```python
from build123d import *

# Parameters (mm, degrees)
F0_W     = 25
F0_H     = 34.675
F0_W_2   = 15.7
F0_H_2   = 27.7
F0_R     = 4.075
F1_DEPTH = 25
F2_R     = 10
F3_R     = 1


with BuildPart() as f1:
    # F0 (on Top) → F1 (new body)
    with BuildSketch(Plane.XY):
        with Locations((0.225, -0.0875)):
            Rectangle(F0_W, F0_H)
        Rectangle(F0_W_2, F0_H_2, mode=Mode.SUBTRACT)
        with BuildLine():
            Line((-12.275, 17.25), (12.725, 17.25))
            Line((12.725, 17.25), (8.530193, 31.366524))
            ThreePointArc((8.530193, 31.366524), (0, 22.836331), (-8.530193, 31.366524))
            Line((-8.530193, 31.366524), (-12.275, 17.25))
        make_face()
        with BuildLine():
            ThreePointArc((-8.530193, 31.366524), (0, 22.836331), (8.530193, 31.366524))
            ThreePointArc((8.530193, 31.366524), (0, 39.896717), (-8.530193, 31.366524))
        make_face()
        with Locations((0, 31.366524)):
            Circle(F0_R, mode=Mode.SUBTRACT)
    extrude(amount=F1_DEPTH)

    # F2
    f2_edges = [f1.edges().sort_by_distance(p)[0] for p in [
        (12.725, 17.25, 12.5),
        (8.530193, 31.366524, 12.5),
        (-8.530193, 31.366524, 12.5),
        (-12.275, 17.25, 12.5),
    ]]
    fillet(f2_edges, radius=F2_R)

    # F3
    f3_edges = [f1.edges().sort_by_distance(p)[0] for p in [
        (12.725, -0.814676, 25),
        (12.620892, 17.234859, 25),
        (0.225, -17.425, 25),
        (10.587354, 24.443688, 25),
        (-12.275, -0.739421, 25),
        (8.631638, 31.192913, 25),
        (-12.191068, 17.239057, 25),
        (-0.040943, 39.896618, 25),
        (-10.370209, 24.430349, 25),
        (-8.612072, 31.208214, 25),
        (7.85, 0, 25),
        (0, -13.85, 25),
        (-7.85, 0, 25),
        (0, 13.85, 25),
        (-4.075, 31.366524, 25),
    ]]
    fillet(f3_edges, radius=F3_R)


solid = f1.part
```
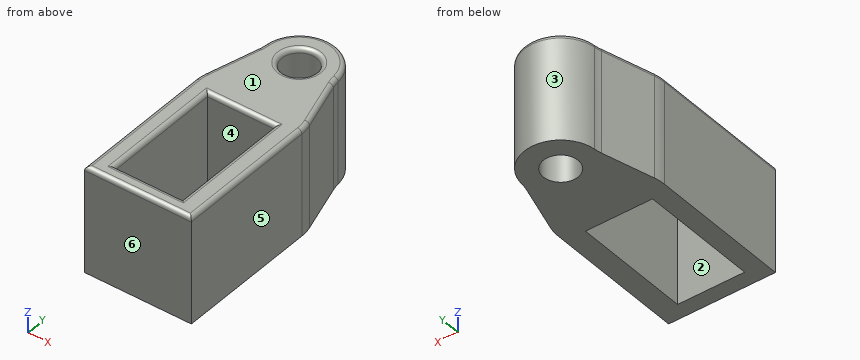
Part model, mm, in its own coordinate system. Face numbers are marked on the shaded views. A direction names the side the tool comes from. Round coordinates to 2 decimals unless told otherwise and drop trailing zeros. Loops run counter-clockwise (first coordinate to the right, second up) from the corner with the lowest first, then second, coordinate; pieces in that order, holes last.
1. Drill centre lines: line 1 along Y through (x, z) = (0, 6.25) (3 decimals); line 2 along X through (y, z) = (13.5, 13.5) (3 decimals); line 3 along Y through (x, z) = (-3.75, 13.5) (3 decimals). Where is each one in solid material? Low to high.
Solutions:
line 1: y = -17.425 to -13.85, 13.85 to 27.292, 35.442 to 39.897
line 2: x = -12.275 to -7.85, 7.85 to 12.725
line 3: y = -17.425 to -13.85, 13.85 to 29.772, 32.961 to 39.028
2. Flat gauge pins, fed straight in: pin 1 (5 mm diameter, centred on x = 4.5, z = 3.5, fed in from +Y); pin 2 (1 mm diameter, centred on x = -3.5, z = 21.5, fed in from +Y); pin 3 (4 mm diameter, centred on y = 21.5, z = 13, fed in from -X); pin 4 (8 mm diameter, centred on x = 1, y = -7, fed in from +Z). Where does each tip first touch, or does it go through?
Solutions:
pin 1: stops at y = 39.66
pin 2: stops at y = 39.35
pin 3: stops at x = -11.68
pin 4: passes through
3. 3-axis set-ups, long thin cutter, end or side, ignore diameter. For the marked faces 1 and 2: which of +Z, -Z, +X, -X, +Y, -Y reach the whole face in a straight line?
Solutions:
face 1: +Z, +X, -X, +Y, -Y
face 2: +Z, -Z
4. Two-plate mould, pull along Y, no slides. Class the marked faces 3, 4, 5 and 6: pulls with the +Y half, pulls with the -Y half, needs draft (parallel to the pull), parting line crosses it, or undercut.
Solutions:
face 3: pulls with the +Y half
face 4: undercut
face 5: needs draft
face 6: pulls with the -Y half
5. Slice it at C-C (x = 3.5). Count the separate pieces of the cut face and the enclosed holes in it, and give its area (3 significant figures).
Solutions:
separate pieces: 3
enclosed holes: 0
area: 616 mm2
6. Slice it at B-B (z = 4.5). Give the cut face in (x, y) (3 decimals).
Solutions:
outline: (-12.275, -17.425) - (12.725, -17.425) - (12.725, 15.796) arc R10 ccw to (12.311, 18.644) - (8.864, 30.243) arc R10 cw to (8.493, 32.161) arc R8.53 ccw to (-8.5, 32.079) arc R10 cw to (-8.8, 30.35) - (-11.941, 18.51) arc R10 ccw to (-12.275, 15.946) - close; hole (-7.85, -13.85) - (7.85, -13.85) - (7.85, 13.85) - (-7.85, 13.85) - close; hole circle Ø8.15 at (0, 31.367)
7. Slice it at A-A (x = 0). Give the cut face in (y, z) (3 decimals).
Solutions:
outline: (-17.425, 0) - (-13.85, 0) - (-13.85, 24) arc R1 ccw to (-14.85, 25) - (-16.425, 25) arc R1 ccw to (-17.425, 24) - close; (13.85, 0) - (27.292, 0) - (27.292, 24) arc R1 ccw to (26.292, 25) - (14.85, 25) arc R1 ccw to (13.85, 24) - close; (35.442, 0) - (39.897, 0) - (39.897, 24) arc R1 ccw to (38.897, 25) - (36.442, 25) arc R1 ccw to (35.442, 24) - close
